For this review, take the finished solid that the model builds, in its own axes (mm). A direction names the side the tool comes from. Give positions to 0.01 mm unless a question says otherwise; leave off trailing zeros. Write each loop counter-clockwise with the first axis right and the second up, starting at its lowest first coordinate (ties: lowest second). Pieces come first, ordered by that corner, then holes.
1) Machinability: for faces 1 (the face through (169, -6, 177.8)), 2 (the face through (336.55, -10, 13)), which of the approach directions +Z, -Z, +X, -X, +Y, -Y give a long, thin tool a straight path to every point of the face, cutting with its end or side? Answer none if there is none.
2) For P1, Ø6.5, axis at x = 101.5, z = 168, coming from the -Y side, flat-tipped, find the tip position at first contact; note if it passes through.
3) Wall thickness on line 1 along Z through (x, y) = (262.5, -10.75); line 2 along Z through (x, y) = (38.1, -8); line 3 along Z through (x, y) = (38.1, -5): over which ranges is each line inside the solid? List them lowest first.
4) We need section C-C on z = 38.1. Give the boundary of the cut face in (x, y).
5) We need section B-B on y = -9.75. Give the boundary of the cut face in (x, z), and give its area (3 significant figures).
6) Draft analysis for pull direction X (two halves, no side actions). For faces 3 (the face through (169, -10, 158.75)), 4 (the face through (169, 0, 90)), 5 (the face through (342.9, -6, 88)), 6 (the face through (0, -6, 88)), state which applies: pulls with the +X half, pulls with the -X half, needs draft (parallel to the pull), parting line crosses it, or undercut.
7) We need section D-D on x = 178.5. Give the boundary of the cut face in (y, z), and give its area (3 significant figures).
8) We need section A-A on x = 38.1. Give the boundary of the cut face in (y, z).
from build123d import *

# Parameters (mm, degrees)
F0_W     = 342.9
F0_H     = 177.8
F1_DEPTH = 12.7
F2_W     = 330.2
F2_H     = 12.7
F3_DEPTH = 6.35
F4_W     = 330.2
F4_H     = 12.7
F5_DEPTH = 6.35
F6_R     = 12.7
F7_DEPTH = 25.4


with BuildPart() as f1:
    # F0 (on Front) → F1 (new body)
    with BuildSketch(Plane.XZ):
        with Locations((171.45, 88.9)):
            Rectangle(F0_W, F0_H)
    extrude(amount=F1_DEPTH)

    # F2 (on face) → F3 (cut)
    with BuildSketch(Plane.XZ.offset(12.7)):
        with Locations((171.45, 12.7)):
            Rectangle(F2_W, F2_H)
    extrude(amount=-F3_DEPTH, mode=Mode.SUBTRACT)

    # F4 (on face) → F5 (cut)
    with BuildSketch(Plane.XZ.offset(12.7)):
        with Locations((171.45, 165.1)):
            Rectangle(F4_W, F4_H)
    extrude(amount=-F5_DEPTH, mode=Mode.SUBTRACT)

    # F6 (on face) → F7 (cut)
    with BuildSketch(Plane(origin=(0, 0, 0), x_dir=(-1, 0, 0), z_dir=(0, 1, 0))):
        with Locations((-38.1, 38.1)):
            Circle(F6_R)
    extrude(amount=-F7_DEPTH, mode=Mode.SUBTRACT)


solid = f1.part
Results list:
1. face 1: +Z, +X, -X, +Y, -Y
1. face 2: -Y
2. P1: stops at y = -6.35
3. line 1: z = 0 to 6.35, 19.05 to 158.75, 171.45 to 177.8
3. line 2: z = 0 to 6.35, 19.05 to 25.4, 50.8 to 158.75, 171.45 to 177.8
3. line 3: z = 0 to 25.4, 50.8 to 177.8
4. outline: (0, -12.7) - (25.4, -12.7) - (25.4, 0) - (0, 0) - close; (50.8, -12.7) - (342.9, -12.7) - (342.9, 0) - (50.8, 0) - close
5. outline: (0, 0) - (342.9, 0) - (342.9, 177.8) - (0, 177.8) - close; hole (6.35, 6.35) - (336.55, 6.35) - (336.55, 19.05) - (6.35, 19.05) - close; hole (6.35, 158.75) - (336.55, 158.75) - (336.55, 171.45) - (6.35, 171.45) - close; hole circle Ø25.4 at (38.1, 38.1)
5. area: 52,100 mm2
6. face 3: undercut
6. face 4: needs draft
6. face 5: pulls with the +X half
6. face 6: pulls with the -X half
7. outline: (-12.7, 0) - (0, 0) - (0, 177.8) - (-12.7, 177.8) - (-12.7, 171.45) - (-6.35, 171.45) - (-6.35, 158.75) - (-12.7, 158.75) - (-12.7, 19.05) - (-6.35, 19.05) - (-6.35, 6.35) - (-12.7, 6.35) - close
7. area: 2,100 mm2
8. outline: (-12.7, 0) - (0, 0) - (0, 25.4) - (-12.7, 25.4) - (-12.7, 19.05) - (-6.35, 19.05) - (-6.35, 6.35) - (-12.7, 6.35) - close; (-12.7, 50.8) - (0, 50.8) - (0, 177.8) - (-12.7, 177.8) - (-12.7, 171.45) - (-6.35, 171.45) - (-6.35, 158.75) - (-12.7, 158.75) - close
